```python
from build123d import *

# Parameters (mm, degrees)
ESBO_O1_W                 = 182
ESBO_O1_H                 = 103.5
RESSALTO_EXTRUS_O1_DEPTH  = 10
ESBO_O2_W                 = 179
ESBO_O2_H                 = 100.5
CORTE_EXTRUS_O1_DEPTH     = 7
ESBO_O4_W                 = 4.8
ESBO_O4_H                 = 9.8
RESSALTO_EXTRUS_O2_DEPTH  = 1
ESPELHAR2_COPY_1_SKETCH_W = 4.8
ESPELHAR2_COPY_1_SKETCH_H = 9.8
ESPELHAR2_COPY_1_DEPTH    = 1
ESBO_O5_W                 = 10
ESBO_O5_H                 = 182
CORTE_EXTRUS_O2_DEPTH     = 3
FILETE3_R                 = 1
FILETE8_R                 = 1
ESBO_O6_R                 = 16
CORTE_EXTRUS_O3_DEPTH     = 10
ESBO_O7_W                 = 25.8
ESBO_O7_H                 = 15
CORTE_EXTRUS_O4_DEPTH     = 10
ESBO_O9_W                 = 15
ESBO_O9_H                 = 15
CORTE_EXTRUS_O5_DEPTH     = 10
ESBO_O10_W                = 7.835934364
ESBO_O10_H                = 20
CORTE_EXTRUS_O6_DEPTH     = 10


with BuildPart() as part:
    # Esboço1 → Ressalto-extrusão1 (new body)
    with BuildSketch(Plane.YZ):
        Rectangle(ESBO_O1_W, ESBO_O1_H)
    extrude(amount=RESSALTO_EXTRUS_O1_DEPTH)

    # Esboço2 → Corte-extrusão1 (cut)
    with BuildSketch(Plane.YZ.offset(10)):
        Rectangle(ESBO_O2_W, ESBO_O2_H)
    extrude(amount=-CORTE_EXTRUS_O1_DEPTH, mode=Mode.SUBTRACT)

    # Esboço4 → Ressalto-extrusão2 (add)
    with BuildSketch(Plane(origin=(0, -89.5, 0), x_dir=(-1, 0, 0), z_dir=(0, 1, 0))):
        with Locations((-7.6, 35.3)):
            Rectangle(ESBO_O4_W, ESBO_O4_H)
    ressalto_extrus_o2 = extrude(amount=RESSALTO_EXTRUS_O2_DEPTH)

    # Espelhar1: Ressalto-extrusão2 across plane
    add(ressalto_extrus_o2.mirror(Plane.XY))

    # Espelhar2: Ressalto-extrusão2 across plane
    add(ressalto_extrus_o2.mirror(Plane.ZX))

    # Espelhar2 copy 1 sketch → Espelhar2 copy 1 (add)
    with BuildSketch(Plane(origin=(0, 89.5, 0), x_dir=(-1, 0, 0), z_dir=(0, -1, 0))):
        with Locations((-7.6, 35.3)):
            Rectangle(ESPELHAR2_COPY_1_SKETCH_W, ESPELHAR2_COPY_1_SKETCH_H)
    extrude(amount=ESPELHAR2_COPY_1_DEPTH)

    # Esboço5 → Corte-extrusão2 (cut)
    with BuildSketch(Plane(origin=(0, 0, -51.75), x_dir=(1, 0, 0), z_dir=(0, 0, -1))):
        with Locations((5, 0)):
            Rectangle(ESBO_O5_W, ESBO_O5_H)
    extrude(amount=-CORTE_EXTRUS_O2_DEPTH, mode=Mode.SUBTRACT)

    # Filete3
    filete3_edges = [part.edges().sort_by_distance(p)[0] for p in [
        (10, 0, 51.75),
        (10, -91, 1.5),
        (0, 0, 51.75),
        (0, -91, 1.5),
        (5, 91, 51.75),
        (0, 91, 1.5),
        (10, 91, 1.5),
        (0, 0, -48.75),
        (5, -91, -48.75),
        (5, 91, -48.75),
    ]]
    fillet(filete3_edges, radius=FILETE3_R)

    # Filete8
    filete8_edges = [part.edges().sort_by_distance(p)[0] for p in [
        (7.6, 88.5, -40.2),
        (5.2, 88.5, -35.3),
        (7.6, 88.5, -30.4),
        (10, 88.5, -35.3),
        (7.6, 88.5, 30.4),
        (5.2, 88.5, 35.3),
        (7.6, 88.5, 40.2),
        (10, 88.5, 35.3),
    ]]
    fillet(filete8_edges, radius=FILETE8_R - 0.0001)  # a hair under: the kernel refuses the full size

    # Esboço6 → Corte-extrusão3 (cut)
    with BuildSketch(Plane(origin=(0, 0, 0), x_dir=(0, -1, 0), z_dir=(-1, 0, 0))):
        with Locations(Location((-71.25, -22.75, 0), (0, 0, 90))):
            Circle(ESBO_O6_R)
    corte_extrus_o3 = extrude(amount=-CORTE_EXTRUS_O3_DEPTH, mode=Mode.SUBTRACT)

    # Espelhar3: Corte-extrusão3 across plane
    add(corte_extrus_o3.mirror(Plane.ZX), mode=Mode.SUBTRACT)

    # Esboço7 → Corte-extrusão4 (cut)
    with BuildSketch(Plane(origin=(0, 0, 0), x_dir=(0, -1, 0), z_dir=(-1, 0, 0))):
        with Locations((0, 28.25)):
            Rectangle(ESBO_O7_W, ESBO_O7_H)
    extrude(amount=-CORTE_EXTRUS_O4_DEPTH, mode=Mode.SUBTRACT)

    # Esboço9 → Corte-extrusão5 (cut)
    with BuildSketch(Plane.YZ.offset(3)):
        with Locations((73.5, 18.25)):
            Rectangle(ESBO_O9_W, ESBO_O9_H)
    extrude(amount=-CORTE_EXTRUS_O5_DEPTH, mode=Mode.SUBTRACT)

    # Esboço10 → Corte-extrusão6 (cut)
    with BuildSketch(Plane.XY.offset(51.75)):
        with Locations((6.917967182, -76)):
            Rectangle(ESBO_O10_W, ESBO_O10_H)
    extrude(amount=-CORTE_EXTRUS_O6_DEPTH, mode=Mode.SUBTRACT)


solid = part.part
```
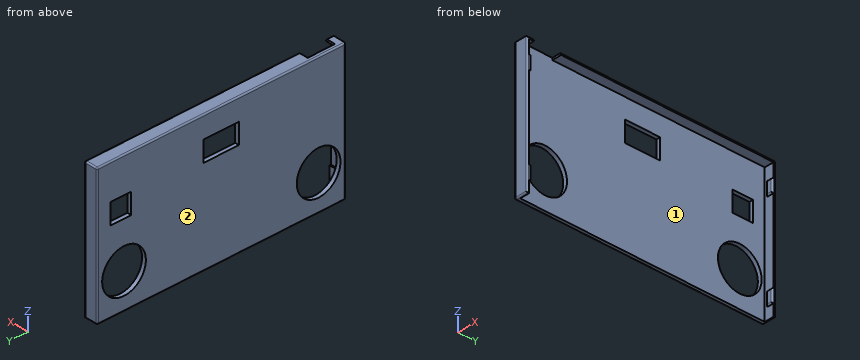
Geometry check sheet. Reference: the model listing, model coordinates, mm. Face numbers are marked on the shaded views. Coordinates: 2 decimals unless noted, no trailing zeros. Write each loop counter-clockwise with the first axis right and the second up, starting at its lowest first coordinate (ties: lowest second). Pieces come first, ordered by that corner, then holes. Notation, with made-up numbers: M 69.5,80 L 84.5,80 A17 ccw 84.5,108 Z; hole C 17.5,87.5 d7. An arc over 180 degrees is marked long. Answer as a JSON object with one key per item and string values.
1. Section check B-B, the plane y = 71.25. Enter the section's corners in (x, z).
Answers below:
{"outline": "M 0,-47.75 A1 ccw 1,-48.75 L 3,-48.75 L 3,-38.75 L 0,-38.75 Z; M 0,-6.75 L 3,-6.75 L 3,10.75 L 0,10.75 Z; M 0,25.75 L 3,25.75 L 3,50.25 L 10,50.25 L 10,50.75 A1 ccw 9,51.75 L 1,51.75 A1 ccw 0,50.75 Z"}
2. Section check A-A, the plane y = -71.25. Enter the section's corners in (x, z), plus the area to 3 significant figures.
Answers below:
{"outline": "M 0,-47.75 A1 ccw 1,-48.75 L 3,-48.75 L 3,-38.75 L 0,-38.75 Z; M 0,-6.75 L 3,-6.75 L 3,51.75 L 1,51.75 A1 ccw 0,50.75 Z", "area": "205 mm²"}
3. Go/stop test with flat-tipped pins: pin 1 Ø1 at (x, y) = (8, -87) entering from -Z; pin 2 Ø3 at (y, z) = (-58, -0.5) entering from +X. Record where each tip stops, or that it passes through.
Answers below:
{"pin 1": "stops at z = 50.25", "pin 2": "stops at x = 3"}
4. Section check D-D, the plane z = -18. Enter the section's corners in (x, y), plus the area to 3 significant figures.
Answers below:
{"outline": "M 0,-90 A1 ccw 1,-91 L 9,-91 A1 ccw 10,-90 L 10,-89.5 L 3,-89.5 L 3,-86.53 L 0,-86.53 Z; M 0,-55.97 L 3,-55.97 L 3,55.97 L 0,55.97 Z; M 0,86.53 L 3,86.53 L 3,89.5 L 10,89.5 L 10,90 A1 ccw 9,91 L 1,91 A1 ccw 0,90 Z", "area": "383 mm²"}
5. Section check C-C, the plane z = 13. Enter the section's corners in (x, y), plus the area to 3 significant figures.
Answers below:
{"outline": "M 0,-90 A1 ccw 1,-91 L 9,-91 A1 ccw 10,-90 L 10,-89.5 L 3,-89.5 L 3,66 L 0,66 Z; M 0,81 L 3,81 L 3,89.5 L 10,89.5 L 10,90 A1 ccw 9,91 L 1,91 A1 ccw 0,90 Z", "area": "521 mm²"}
6. Scan lines: L1, parallel to Y at x = 1.05, z = -22.75; L2, parallel to Y at x = 4.5, z = 7; L3, parallel to Z at x = 0.95, y = -71.25. Record each from-to range of solid material in increasing order.
Answers below:
{"L1": "y = -91 to -87.25, -55.25 to 55.25, 87.25 to 91", "L2": "y = -91 to -89.5, 89.5 to 91", "L3": "z = -48.75 to -38.75, -6.75 to 51.75"}
7. Draft check along Y on the marked faces 1 and 2. Enter one of: released by +Y, released by -Y, zero draft, split by the parting line, or undercut.
Answers below:
{"face 1": "undercut", "face 2": "zero draft"}
